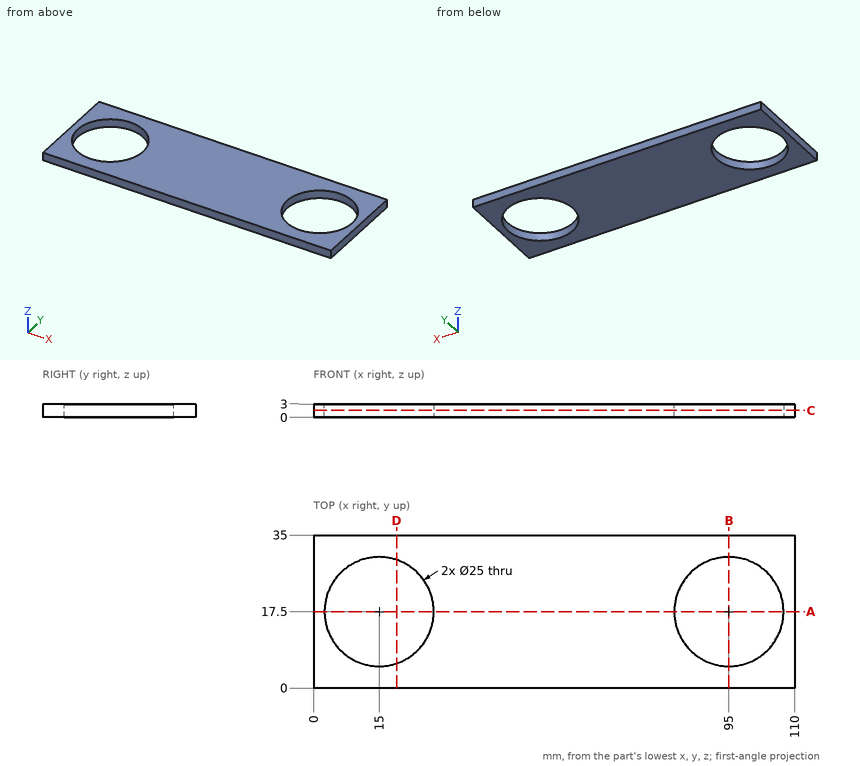
Geometry check sheet. Reference: drawing and pictorial views, mm from the part's lowest x, y, z. Coordinates: 2 decimals unless noted, no trailing zeros. Write each loop counter-clockwise with the first axis right and the second up, starting at its lowest first coordinate (ties: lowest second). Pieces come first, ordered by that corner, then holes.
Item 1: Cross-section at D-D on x = 19. Record the boundary of the cut face in (y, z).
Numbers:
outline: (0, 0) - (5.66, 0) - (5.66, 3) - (0, 3) - close; (29.34, 0) - (35, 0) - (35, 3) - (29.34, 3) - close
Item 2: Depth check by flat-ended pin: pin 1 Ø15 at (x, y) = (15, 17.5) entering from -Z. Enter the tip coordinate at first touch or a pass-through.
Numbers:
pin 1: passes through
Item 3: Cross-section at A-A on y = 17.5. Record the boundary of the cut face in (x, z).
Numbers:
outline: (0, 0) - (2.5, 0) - (2.5, 3) - (0, 3) - close; (27.5, 0) - (82.5, 0) - (82.5, 3) - (27.5, 3) - close; (107.5, 0) - (110, 0) - (110, 3) - (107.5, 3) - close
Item 4: Cross-section at C-C on z = 1.55. Record the boundary of the cut face in (x, y), then the cut area to 3 significant figures.
Numbers:
outline: (0, 0) - (110, 0) - (110, 35) - (0, 35) - close; hole circle Ø25 at (15, 17.5); hole circle Ø25 at (95, 17.5)
area: 2,870 mm2
Item 5: Cross-section at B-B on x = 95. Record the boundary of the cut face in (y, z), then the cut area to 3 significant figures.
Numbers:
outline: (0, 0) - (5, 0) - (5, 3) - (0, 3) - close; (30, 0) - (35, 0) - (35, 3) - (30, 3) - close
area: 30.0 mm2
Item 6: Scan lines: probe 1 along Y at (x, z) = (95, 1.6); probe 2 along X at (y, z) = (26, 2.55); probe 3 along X at (y, z) = (10.5, 2.1). Record each from-to range of solid material in increasing order.
Numbers:
probe 1: y = 0 to 5, 30 to 35
probe 2: x = 0 to 5.83, 24.17 to 85.83, 104.17 to 110
probe 3: x = 0 to 4.64, 25.36 to 84.64, 105.36 to 110
